Read the model definition and answer for the solid it produces. Units are mm, in the model's axes. A direction names the side the tool comes from. Coordinates: 2 decimals unless noted, no trailing zeros. Write each loop counter-clockwise with the first axis right and the second up, starting at its lowest first coordinate (ties: lowest second). Pieces come first, ordered by that corner, then holes. Notation, with made-up numbers: (52.25, 78) - (84.25, 78) arc R17 cw to (84.25, 95) - close; hole circle Ø7 at (11, 76). An arc over 180 degrees is marked (long way). Use a Markdown table: item, result.
Autodesk Inventor part; units mm, degrees
ref_plane "Work Plane1" through (0, 0, 29.25) normal (0, 0, 1) x (1, 0, 0)
ref_plane "YZ Plane" through (0, 0, 0) normal (1, 0, 0) x (0, 1, 0)
ref_plane "XZ Plane" through (0, 0, 0) normal (0, 1, 0) x (-1, 0, 0)
sketch "Sketch1" plane through (0, 0, 0) normal (0, 1, 0) x (-1, 0, 0)
  line L0 (3, 20.25) -> (-3, 20.25)
  line L1 (-3, 20.25) -> (-3, -20.25)
  line L2 (-3, -20.25) -> (3, -20.25)
  line L3 (3, -20.25) -> (3, 20.25)
  line L4 (3, 20.25) -> (-3, -20.25) construction
  line L5 (-3, 20.25) -> (3, -20.25) construction
  point P0 (0, 0)
  dimension "d0" = 6
  dimension "d1" = 40.5
extrude "Extrusion1" add sketch "Sketch1" along normal blind 10
fillet "Fillet1" radius 8 1 edges at (0, 0, -20.25)
sketch "Sketch2" plane through (0, 10, 0) normal (0, 1, 0) x (1, 0, 0)
  line L0 (3, 20.25) -> (-3, 20.25) construction
  line L1 (0, 20.25) -> (0, -24.25) construction
  circle A0 centre (0, -24.25) radius 5
  point P0 (0, 0)
  dimension "d5" = 44.5
  dimension "d6" = 10
extrude "Extrusion2" add sketch "Sketch2" along normal blind 14.5 and the other way blind 15
sketch "Sketch3" plane through (0, 0, 0) normal (0, -1, 0) x (1, 0, 0)
  line L0 (3, -20.25) -> (-3, -20.25) construction
  line L1 (0, -20.25) -> (0, 3.75) construction
  circle A0 centre (0, 3.75) radius 5
  point P0 (0, 0)
  dimension "d11" = 24
  dimension "d12" = 10
extrude "Extrusion3" add sketch "Sketch3" along normal blind 25.5 and the other way blind 7
sketch "Sketch4" plane through (0, 10, 0) normal (0, 1, 0) x (1, 0, 0)
  line L0 (-3, 20.25) -> (3, 20.25) construction
  line L1 (0, 20.25) -> (0, 12.25) construction
  line L2 (-12.5, 4.25) -> (12.5, 4.25)
  line L3 (12.5, 4.25) -> (12.5, 20.25)
  line L4 (12.5, 20.25) -> (-12.5, 20.25)
  line L5 (-12.5, 20.25) -> (-12.5, 4.25)
  line L6 (-12.5, 4.25) -> (12.5, 20.25) construction
  line L7 (12.5, 4.25) -> (-12.5, 20.25) construction
  point P0 (0, 0)
  dimension "d17" = 8
  dimension "d18" = 25
extrude "Extrusion4" add sketch "Sketch4" along normal blind 6 and the other way blind 0.5
sketch "Sketch5" plane through (0, 16, 0) normal (0, 1, 0) x (1, 0, 0)
  line L0 (-3, 20.25) -> (3, 20.25) construction
  line L1 (0, 20.25) -> (0, 12.25) construction
  line L2 (0, 12.25) -> (-8, 12.25) construction
  circle A0 centre (-8, 12.25) radius 1.6
  circle A1 centre (8, 12.25) radius 1.6
  point P0 (0, 0)
  dimension "d23" = 8
  dimension "d24" = 8
  dimension "d25" = 3.2
extrude "Extrusion5" cut sketch "Sketch5" against normal through all
sketch "Sketch6" plane through (0, 24.5, 24.25) normal (0, 1, 0) x (1, 0, 0)
  circle A0 centre (0, 0) radius 2.5
  point P0 (0, 24.25)
  dimension "d28" = 5
extrude "Extrusion6" cut sketch "Sketch6" against normal through all
ref_plane "Work Plane1" through (0, 0, 29.25) normal (0, 0, 1) x (1, 0, 0)
sketch "Sketch8" plane through (0, 0, 29.25) normal (0, 0, 1) x (1, 0, 0)
  line L0 (5, 24.5) -> (-5, 24.5)
  line L1 (0, 24.5) -> (0, 9.75)
  circle A0 centre (0, 9.75) radius 0.8
  point P0 (0, 0)
  dimension "d39" = 14.75
  dimension "d40" = 1.6
hole "Hole2" at (0, 9.75, 29.25) direction (0, 0, -1) diameter 1.6 end up to surface countersink diameter 1.7 countersink angle 45
properties part number "Supporto SX"
(1) A cutting plane is placed at D-D, the plane x = 8. Write down the section's boundary in (y, z).
Report:
| item | result |
|---|---|
| outline | (9.5, -20.25) - (16, -20.25) - (16, -13.85) - (9.5, -13.85) - close; (9.5, -10.65) - (16, -10.65) - (16, -4.25) - (9.5, -4.25) - close |
(2) Each of these flat-tipped pins is pushed along its axis until it touches: P1, Ø1.6, axis at x = 3.5, z = 4.5, coming from the +Y side; P2, Ø1, axis at x = -4, z = 3, coming from the +Y side; P3, Ø6, axis at x = 0, z = 24.25, coming from the +Y side; P4, Ø1.8, axis at x = 0.5, z = 16, coming from the -Y side. Where does it stop, or does it pass through?
Report:
| item | result |
|---|---|
| P1 | stops at y = 10 |
| P2 | stops at y = 7 |
| P3 | stops at y = 24.5 |
| P4 | stops at y = 0 |
(3) A cutting plane is placed at A-A, the plane y = 14. Write down the section's boundary in (x, z).
Report:
| item | result |
|---|---|
| outline | (-12.5, -20.25) - (12.5, -20.25) - (12.5, -4.25) - (-12.5, -4.25) - close; circle Ø10 at (0, 24.25); hole circle Ø3.2 at (-8, -12.25); hole circle Ø5 at (0, 24.25); hole circle Ø3.2 at (8, -12.25) |
(4) A cutting plane is placed at B-B, the plane x = 0. Write down the section's boundary in (y, z), and give its area (3 significant figures).
Report:
| item | result |
|---|---|
| outline | (-25.5, -1.25) - (0, -1.25) - (0, -12.25) arc R8 ccw to (8, -20.25) - (16, -20.25) - (16, -4.25) - (10, -4.25) - (10, 19.25) - (24.5, 19.25) - (24.5, 21.75) - (-5, 21.75) - (-5, 19.25) - (0, 19.25) - (0, 8.75) - (-25.5, 8.75) - close; (-5, 26.75) - (8.95, 26.75) - (8.95, 29.13) - (8.9, 29.25) - (-5, 29.25) - close; (10.55, 26.75) - (24.5, 26.75) - (24.5, 29.25) - (10.6, 29.25) - (10.55, 29.13) - close |
| area | 876 mm² |
(5) For faces 1 (the flat face through (0, -25.5, 4)), 2 (the cylindrical face through (6.82, 12.8, -13.33)), 3 (the flat face through (-4, 7, 4)), 4 (the cylindrical face through (-4.995, -9.478, 3.97)), 5 (the flat face through (8, 9.5, -14)), determine the directions among +Z, -Z, +X, -X, +Y, -Y from which every point of the face is accessible in a straight line to the end or side of a thin tool.
Report:
| item | result |
|---|---|
| face 1 | +Z, -Z, +X, -X, -Y |
| face 2 | +Y, -Y |
| face 3 | -Z, -X, +Y |
| face 4 | -Y |
| face 5 | -Z, +X, -Y |
(6) The mould has two halves that part along Z. Classify faces 6 (the cylindrical face through (-0.042, 2.406, -17.969)), 7 (the flat face through (3, 7.2, 0.3)), 8 (the flat face through (2, 24.5, 26)): pulls with the +Z half, pulls with the -Z half, needs draft (parallel to the pull), parting line crosses it, or undercut.
Report:
| item | result |
|---|---|
| face 6 | pulls with the -Z half |
| face 7 | undercut |
| face 8 | needs draft |
(7) A cutting plane is placed at C-C, the plane z = 24.25. Write down the section's boundary in (x, y).
Report:
| item | result |
|---|---|
| outline | (-5, -5) - (-2.5, -5) - (-2.5, 24.5) - (-5, 24.5) - close; (2.5, -5) - (5, -5) - (5, 24.5) - (2.5, 24.5) - close |
(8) Straight lines are drawn through the part: L1, parallel to X at y = 14.5, z = -12.25; L2, parallel to Z at x = 0, y = 10.75; L3, parallel to Z at x = 8, y = 14.5. For each, find the intervals that lie inside material, in ascending order.
Report:
| item | result |
|---|---|
| L1 | x = -12.5 to -9.6, -6.4 to 6.4, 9.6 to 12.5 |
| L2 | z = -20.25 to -4.25, 19.25 to 21.75, 26.75 to 29.25 |
| L3 | z = -20.25 to -13.85, -10.65 to -4.25 |
